from build123d import *

# Parameters (mm, degrees)
F0_W     = 101.6
F0_H     = 76.2
F1_DEPTH = 152.4
F2_W     = 76.2
F2_H     = 25.4
F3_DEPTH = 50.8
F4_R     = 5.08


with BuildPart() as f1:
    # F0 (on Top) → F1 (new body)
    with BuildSketch(Plane.XY):
        with Locations((0.049565, -1.278337)):
            Rectangle(F0_W, F0_H)
    extrude(amount=F1_DEPTH)

    # F2 (on face) → F3 (cut)
    with BuildSketch(Plane.XZ.offset(39.378337)):
        with Locations((0.049565, 129.54)):
            Rectangle(F2_W, F2_H)
        with Locations((0.049565, 93.98)):
            Rectangle(F2_W, F2_H)
        with Locations((0.049565, 58.42)):
            Rectangle(F2_W, F2_H)
        with Locations((0.049565, 22.86)):
            Rectangle(F2_W, F2_H)
    extrude(amount=-F3_DEPTH, mode=Mode.SUBTRACT)

    # F4
    f4_edges = [f1.edges().sort_by_distance(p)[0] for p in [
        (50.849565, -1.278337, 152.4),
        (0.049565, 36.821663, 152.4),
        (-50.750435, -1.278337, 152.4),
        (0.049565, -39.378337, 152.4),
        (50.849565, -39.378337, 76.2),
        (50.849565, 36.821663, 76.2),
        (50.849565, -1.278337, 0),
        (-50.750435, 36.821663, 76.2),
        (-50.750435, -39.378337, 76.2),
        (-50.750435, -1.278337, 0),
    ]]
    fillet(f4_edges, radius=F4_R)


solid = f1.part
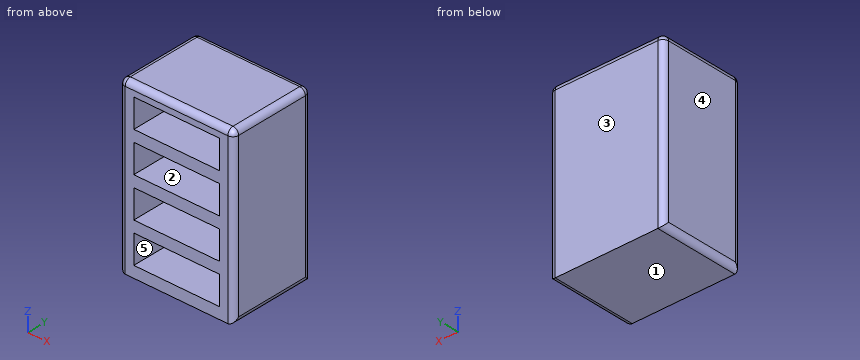
Part model, mm, in its own coordinate system. Face numbers are marked on the shaded views. A direction names the side the tool comes from. Coordinates: 2 decimals unless noted, no trailing zeros. Write each loop counter-clockwise with the first axis right and the second up, starting at its lowest first coordinate (ties: lowest second). Pieces come first, ordered by that corner, then holes. Notation, with made-up numbers: (51.5, -38) - (90.5, -38) arc R4 cw to (90.5, -33) - close; hole circle Ø5 at (-29, 57). An arc over 180 degrees is marked (long way). Put each result on its own line as item: value.
1. Band-saw the part on B-B (x = 23). Write the cut outline in (y, z).
Final values:
outline: (-39.38, 0) - (36.82, 0) - (36.82, 147.32) arc R5.08 ccw to (31.74, 152.4) - (-34.3, 152.4) arc R5.08 ccw to (-39.38, 147.32) - (-39.38, 142.24) - (11.42, 142.24) - (11.42, 116.84) - (-39.38, 116.84) - (-39.38, 106.68) - (11.42, 106.68) - (11.42, 81.28) - (-39.38, 81.28) - (-39.38, 71.12) - (11.42, 71.12) - (11.42, 45.72) - (-39.38, 45.72) - (-39.38, 35.56) - (11.42, 35.56) - (11.42, 10.16) - (-39.38, 10.16) - close
2. Band-saw the part on C-C (z = 24). Write the cut outline in (x, y), then the cut area to 3 significant figures.
Final values:
outline: (-50.75, -34.3) arc R5.08 ccw to (-45.67, -39.38) - (-38.05, -39.38) - (-38.05, 11.42) - (38.15, 11.42) - (38.15, -39.38) - (45.77, -39.38) arc R5.08 ccw to (50.85, -34.3) - (50.85, 31.74) arc R5.08 ccw to (45.77, 36.82) - (-45.67, 36.82) arc R5.08 ccw to (-50.75, 31.74) - close
area: 3,850 mm²
3. Band-saw the part on A-A (y = -24.5). Write the cut outline in (x, z), then the cut area to 3 significant figures.
Final values:
outline: (-50.75, 5.08) arc R5.08 ccw to (-45.67, 0) - (45.77, 0) arc R5.08 ccw to (50.85, 5.08) - (50.85, 147.32) arc R5.08 ccw to (45.77, 152.4) - (-45.67, 152.4) arc R5.08 ccw to (-50.75, 147.32) - close; hole (-38.05, 10.16) - (38.15, 10.16) - (38.15, 35.56) - (-38.05, 35.56) - close; hole (-38.05, 45.72) - (38.15, 45.72) - (38.15, 71.12) - (-38.05, 71.12) - close; hole (-38.05, 81.28) - (38.15, 81.28) - (38.15, 106.68) - (-38.05, 106.68) - close; hole (-38.05, 116.84) - (38.15, 116.84) - (38.15, 142.24) - (-38.05, 142.24) - close
area: 7,720 mm²
4. Flat gauge pins, fed straight in: pin 1 Ø15 at (x, y) = (2.5, -16.5) entering from -Z; pin 2 Ø7.5 at (x, z) = (8, 22) entering from -Y. Where does each tip first touch, or does it go through?
Final values:
pin 1: stops at z = 0
pin 2: stops at y = 11.42
5. 3-axis set-ups, long thin cutter, end or side, ignore diameter. For the marked faces 1 and 2: which of +Z, -Z, +X, -X, +Y, -Y reach the whole face in a straight line?
Final values:
face 1: -Z, +X, -X, +Y, -Y
face 2: -Y
6. Two-plate mould, pull along X, no slides. Class the marked faces 3, 4 and 5: +X half, -X half, draft (parallel to the pull), parting line (faces both ways), or undercut.
Final values:
face 3: draft
face 4: -X half
face 5: undercut
7. Probe line 1 along Z through (x, y) = (1, 0.5); line 2 along X through (y, z) = (11, 17); line 3 along Y through (x, z) = (-24, 124.5). List the from-to ranges inside material, lowest first. Write a range as [from, to].
Final values:
line 1: z = [0, 10.16], [35.56, 45.72], [71.12, 81.28], [106.68, 116.84], [142.24, 152.4]
line 2: x = [-50.75, -38.05], [38.15, 50.85]
line 3: y = [11.42, 36.82]
